Read the model definition and answer for the solid it produces. Units are mm, in the model's axes. A direction names the side the tool comes from. Coordinates: 2 decimals unless noted, no trailing zeros. Write each loop counter-clockwise with the first axis right and the second up, starting at its lowest first coordinate (ties: lowest second). Pieces come first, ordered by that corner, then holes.
Item 1: Section B-B (y = 15.5) is taken. Give the vertices of the cut face in (x, z).
Item 2: A tool of negligible diameter and unlimited length cuts with its end or side. For faces 3 (the face through (-98.285, 4.121, 2.507)), 4 (the face through (-92.24, 40.7, 6.77)), 5 (the face through (-58, 2.22, 6)), 6 (the face through (-60.647, 41, 6)), 7 (the face through (-73, -2.78, 1)), from which of +Z, -Z, +X, -X, +Y, -Y can it reach the whole face along a straight path? Write none if from no direction.
Item 3: Determine the mould class of faces 1 (the face through (-92.24, 3.7, 6.77)), 2 (the face through (-58, 39.22, 6)) for opening direction X: released by +X, released by -X, zero draft, split by the parting line, or undercut.
Item 4: Section A-A (z = 6.25) is taken. State how many separate pieces and enclosed holes the cut face has, then the cut area to 3 significant figures.
Item 5: Section C-C (x = -43) is taken. Give the vertices of the cut face in (y, z).
Item 6: Each of these flat-tipped pins is pushed along its axis until it touches: P1, Ø6.5, axis at x = -77.5, y = 3.5, coming from the +Z side; P2, Ø2, axis at x = -31.5, z = 6.5, coming from the +Y side; P3, Ø12, axis at x = -55, y = 31, coming from the -Z side; P4, Ø3, axis at x = -58, z = 7, coming from the -Y side. Where does it stop, or does it pass through?
Item 7: Straight lines are drawn through the part: probe 1 along Y at (x, z) = (-92, 4.5); probe 2 along Z at (x, y) = (-88.5, 36). For each, find the intervals that lie inside material, in ascending order.
from build123d import *

# Parameters (mm, degrees)
SKETCH_1_W          = 89
SKETCH_1_H          = 40
EXTRUDE_1_DEPTH     = 3
SKETCH_2_W          = 32.5
SKETCH_2_H          = 3
EXTRUDE_2_DEPTH     = 6.5
SKETCH_3_R          = 2.4
CUT_EXTRUDE_1_DEPTH = 100
SKETCH_5_W          = 3
SKETCH_5_H          = 5
EXTRUDE_3_DEPTH     = 89
SKETCH_7_W          = 11.5
SKETCH_7_H          = 50
CUT_EXTRUDE_2_DEPTH = 6.5
SKETCH_8_R          = 1.62
CUT_EXTRUDE_3_DEPTH = 127.662192681
SKETCH_9_R          = 3
CUT_EXTRUDE_4_DEPTH = 1


with BuildPart() as part:
    # 草图1 → 凸台-拉伸1 (new body)
    with BuildSketch(Plane.XY):
        with Locations((-72.64664311, 22.219964664)):
            Rectangle(SKETCH_1_W, SKETCH_1_H)
    extrude(amount=EXTRUDE_1_DEPTH)

    # 草图2 → 凸台-拉伸2 (add)
    with BuildSketch(Plane.XY.offset(3)):
        with Locations((-100.89664311, 40.719964664)):
            Rectangle(SKETCH_2_W, SKETCH_2_H)
        with Locations((-100.89664311, 3.719964664)):
            Rectangle(SKETCH_2_W, SKETCH_2_H)
        with Locations((-44.39664311, 40.719964664)):
            Rectangle(SKETCH_2_W, SKETCH_2_H)
        with Locations((-44.39664311, 3.719964664)):
            Rectangle(SKETCH_2_W, SKETCH_2_H)
    extrude(amount=EXTRUDE_2_DEPTH)

    # 草图3 → 切除-拉伸1 (cut)
    with BuildSketch(Plane(origin=(0, 2.219964664, 0), x_dir=(-1, 0, 0), z_dir=(0, -1, 0))):
        with Locations(Location((111.89664311, -6.25, 0), (0, 0, 90))):
            Circle(SKETCH_3_R)
        with Locations(Location((89.89664311, -6.25, 0), (0, 0, 90))):
            Circle(SKETCH_3_R)
        with Locations(Location((55.39664311, -6.25, 0), (0, 0, 90))):
            Circle(SKETCH_3_R)
        with Locations(Location((33.39664311, -6.25, 0), (0, 0, 90))):
            Circle(SKETCH_3_R)
    extrude(amount=-CUT_EXTRUDE_1_DEPTH, mode=Mode.SUBTRACT)

    # 草图5 → 凸台-拉伸3 (add)
    with BuildSketch(Plane.ZY.offset(117.14664311)):
        with Locations((1.5, 44.719964664)):
            Rectangle(SKETCH_5_W, SKETCH_5_H)
        with Locations((1.5, -0.280035336)):
            Rectangle(SKETCH_5_W, SKETCH_5_H)
    extrude(amount=-EXTRUDE_3_DEPTH)

    # 草图7 → 切除-拉伸2 (cut)
    with BuildSketch(Plane.XY.offset(9.5)):
        with Locations((-100.89664311, 22.219964664)):
            Rectangle(SKETCH_7_W, SKETCH_7_H)
        with Locations((-44.39664311, 22.219964664)):
            Rectangle(SKETCH_7_W, SKETCH_7_H)
    extrude(amount=-CUT_EXTRUDE_2_DEPTH, mode=Mode.SUBTRACT)

    # 草图8 → 切除-拉伸3 (cut, through all)
    with BuildSketch(Plane(origin=(0, 0, 0), x_dir=(-1, 0, 0), z_dir=(0, 0, -1))):
        with Locations((101.14664311, 41.219964664)):
            Circle(SKETCH_8_R)
        with Locations((101.14664311, 3.219964664)):
            Circle(SKETCH_8_R)
        with Locations((76.14664311, 41.219964664)):
            Circle(SKETCH_8_R)
        with Locations((76.14664311, 3.219964664)):
            Circle(SKETCH_8_R)
    extrude(amount=-CUT_EXTRUDE_3_DEPTH, mode=Mode.SUBTRACT)

    # 草图9 → 切除-拉伸4 (cut)
    with BuildSketch(Plane.XY.offset(3)):
        with Locations((-76.14664311, 41.219964664)):
            Circle(SKETCH_9_R)
        with Locations((-101.14664311, 41.219964664)):
            Circle(SKETCH_9_R)
        with Locations((-101.14664311, 3.219964664)):
            Circle(SKETCH_9_R)
        with Locations((-76.14664311, 3.219964664)):
            Circle(SKETCH_9_R)
    extrude(amount=-CUT_EXTRUDE_4_DEPTH, mode=Mode.SUBTRACT)


solid = part.part
Established:
1. outline: (-117.15, 0) - (-28.15, 0) - (-28.15, 3) - (-117.15, 3) - close
2. face 3: +Z
2. face 4: +Y, -Y
2. face 5: +Z, +X, -X, -Y
2. face 6: +Z, +Y, -Y
2. face 7: +Z, -Z, +X, -X, -Y
3. face 1: undercut
3. face 2: zero draft
4. separate pieces: 16
4. enclosed holes: 0
4. area: 137 mm2
5. outline: (-2.78, 0) - (47.22, 0) - (47.22, 3) - (-2.78, 3) - close
6. P1: stops at z = 3
6. P2: stops at y = 42.22
6. P3: stops at z = 0
6. P4: stops at y = 2.22
7. probe 1: y = 2.22 to 5.22, 39.22 to 42.22
7. probe 2: z = 0 to 3
